from build123d import *

# Parameters (mm, degrees)
BOSS_EXTRU_1_DEPTH      = 8
ESQUISSE2_R             = 7.5
BOSS_EXTRU_2_DEPTH      = 2
ENL_V_MAT_EXTRU_1_REACH = 16.577


with BuildPart() as part:
    # Esquisse1 → Boss.-Extru.1 (new body)
    with BuildSketch(Plane.XY):
        Polygon((0, 7.390083446), (-6.4, 3.695041723), (-6.4, -3.695041723), (0, -7.390083446), (6.4, -3.695041723), (6.4, 3.695041723), align=None)
    extrude(amount=BOSS_EXTRU_1_DEPTH)

    # Esquisse2 → Boss.-Extru.2 (add)
    with BuildSketch(Plane.XY.offset(8)):
        Circle(ESQUISSE2_R)
    extrude(amount=BOSS_EXTRU_2_DEPTH)

    # Esquisse3 → Enlèv. mat.-Extru.1 (cut, up to next)
    with BuildSketch(Plane(origin=(0, 0, 0), x_dir=(-1, 0, 0), z_dir=(0, 0, -1)), mode=Mode.PRIVATE) as enl_v_mat_extru_1_sk1:
        with BuildLine():
            Line((-1, 1.374772708), (-1, -1.374772708))
            ThreePointArc((-1, -1.374772708), (0.53749696, -1.612791684), (1.624807681, -0.5))
            Line((1.624807681, -0.5), (8.490964129, -0.5))
            Line((8.490964129, -0.5), (8.490964129, 0.5))
            Line((8.490964129, 0.5), (1.624807681, 0.5))
            ThreePointArc((1.624807681, 0.5), (0.53749696, 1.612791684), (-1, 1.374772708))
        make_face()
    enl_v_mat_extru_1_tool1 = extrude(enl_v_mat_extru_1_sk1.sketch, amount=-ENL_V_MAT_EXTRU_1_REACH, mode=Mode.PRIVATE) & part.part
    add(enl_v_mat_extru_1_tool1.solids().sort_by_distance((-2.500554, 0, 0))[0], mode=Mode.SUBTRACT)


solid = part.part
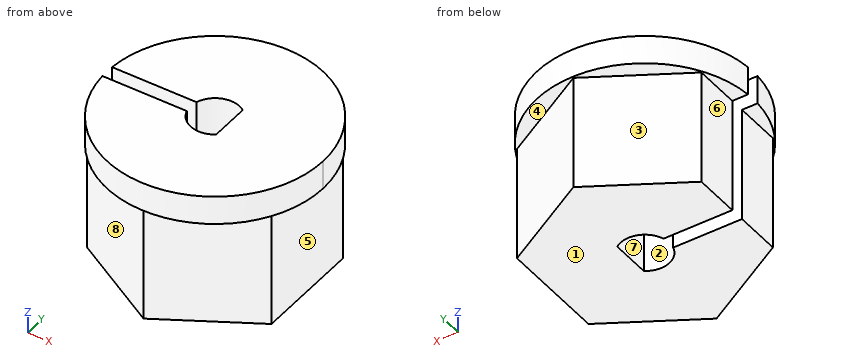
Can you work these out from the model? Positions are in its coordinate system, mm. Face numbers are marked on the shaded views. A direction names the side the tool comes from. Give positions to 0.01 mm unless a question says otherwise; leave off trailing zeros. Order: outer loops, then holes, each group sorted by start corner. A loop starts at its lowest first (then second) coordinate and runs counter-clockwise, first axis right, second up. Notation, with made-up numbers: M -17.5,87.5 L 6.5,87.5 A22 cw 6.5,113.5 Z; hole C -9.75,58 d6. An arc over 180 degrees is marked long. One line per item, written item: value.
Item 1: If we section it at C-C on z = 6: Write out the boundary of the cut face in (x, y), and give its area (3 significant figures).
Verdict:
outline: M -6.4,-3.7 L 0,-7.39 L 6.4,-3.7 L 6.4,3.7 L 0,7.39 L -6.4,3.7 L -6.4,0.5 L -1.62,0.5 A1.7 cw 1,1.37 L 1,-1.37 A1.7 cw -1.62,-0.5 L -6.4,-0.5 Z
area: 129 mm2
Item 2: If we section it at D-D on x = 4: Write out the boundary of the cut face in (y, z), and give its area (3 significant figures).
Verdict:
outline: M -6.34,8 L -5.08,8 L -5.08,0 L 5.08,0 L 5.08,8 L 6.34,8 L 6.34,10 L -6.34,10 Z
area: 107 mm2
Item 3: If we section it at B-B on y = -0.75: Write out the boundary of the cut face in (x, z), and give its area (3 significant figures).
Verdict:
outline: M -7.46,8 L -6.4,8 L -6.4,0 L -1.53,0 L -1.53,10 L -7.46,10 Z; M 1,0 L 6.4,0 L 6.4,8 L 7.46,8 L 7.46,10 L 1,10 Z
area: 107 mm2
Item 4: If we section it at A-A on x = -4: Write out the boundary of the cut face in (y, z), and give its area (3 significant figures).
Verdict:
outline: M -6.34,8 L -5.08,8 L -5.08,0 L -0.5,0 L -0.5,10 L -6.34,10 Z; M 0.5,0 L 5.08,0 L 5.08,8 L 6.34,8 L 6.34,10 L 0.5,10 Z
area: 96.7 mm2
Item 5: If we mould it in two halves opening along Y, with no side actions, what happens to the marked faces 1, 2 and 3? For each: pulls with the +Y half, pulls with the -Y half, needs draft (parallel to the pull), parting line crosses it, or undercut.
Verdict:
face 1: needs draft
face 2: undercut
face 3: pulls with the +Y half
Item 6: Please list where these lines run through material, in increasing order: line 1 (X direction, y = 3.5, z = 7.5); line 2 (Y direction, x = -6, z = 3.5); line 3 (Y direction, x = -1, z = 8.5).
Verdict:
line 1: -6.4 to 6.4
line 2: -3.93 to -0.5, 0.5 to 3.93
line 3: -7.43 to -1.37, 1.37 to 7.43
Item 7: For pin 1 (3.5 mm diameter, centred on y = -1.5, z = 6, fed in from -X); pin 2 (5 mm diameter, centred on x = -2, z = 6, fed in from +Y); pin 3 (3 mm diameter, centred on x = 5, z = 8.5, fed in from +Y), each with a flat end and sliding along its axis, tell me the tip position at first contact or that it passes through.
Verdict:
pin 1: x = -6.4
pin 2: y = 7.48
pin 3: y = 6.63
Item 8: For the marked faces 4, 5, 6, 7 and 8, which set-ups out of +Z, -Z, +X, -X, +Y, -Y let a thin tool reach every point of the face, with its end or its side?
Verdict:
face 4: -Z
face 5: -Z, +X, +Y, -Y
face 6: -Z, -X, +Y, -Y
face 7: +Z, -Z
face 8: -Z, -X, -Y
